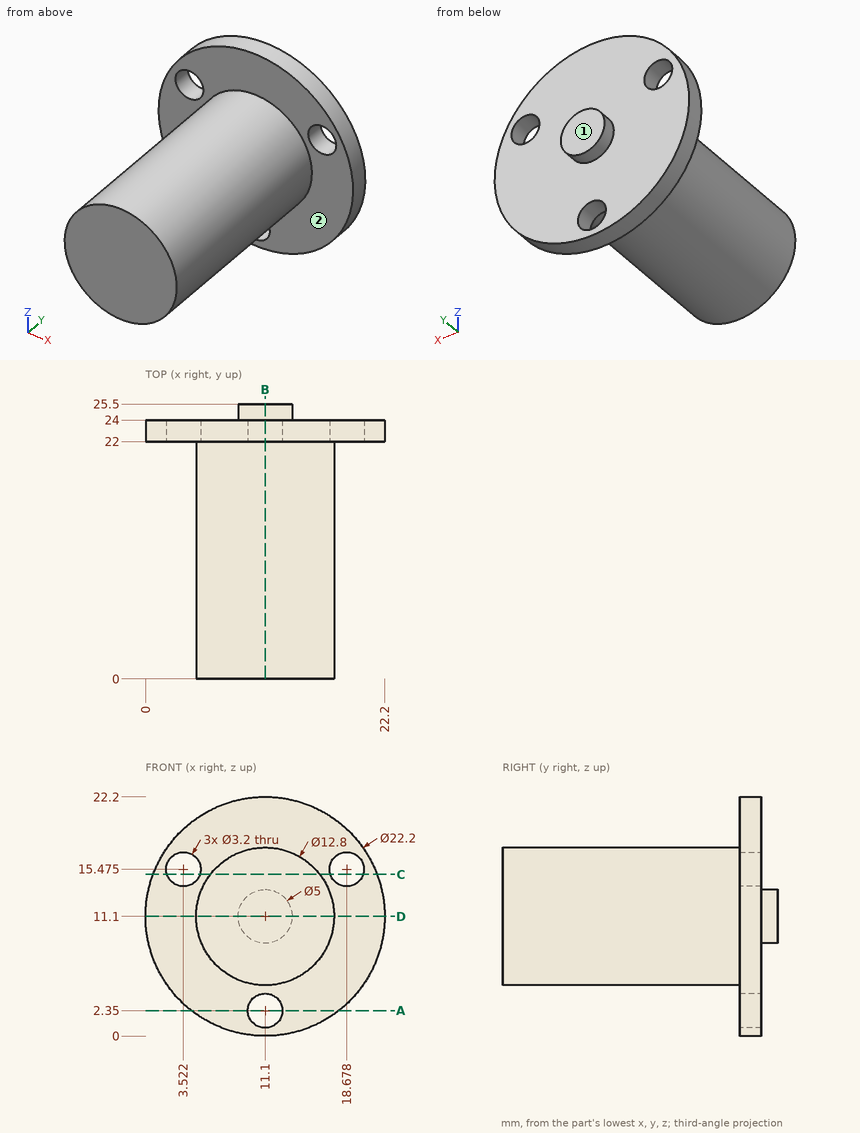
Drawing for the job (mm, zero at the part's lowest x, y, z). A direction names the side the tool comes from. Round coordinates to 2 decimals unless told otherwise and drop trailing zeros. Order: outer loops, then holes, each group sorted by start corner. A loop starts at its lowest first (then second) coordinate and runs counter-clockwise, first axis right, second up. Notation, with made-up numbers: (52, 62) -> (79, 62) arc R22 ccw to (79, 79) -> close; hole circle Ø5 at (85.5, 15.5). An arc over 180 degrees is marked (long way). Write item = value, one per line. Start each with the question number.
(1) Which spindle directions (+Z, -Z, +X, -X, +Y, -Y) get a long thin tool onto all of the face, cutting with end or side? Do the marked faces 1 and 2. Say none if no direction does.
(2) Pin check, flat tips, straight feed: P1, Ø5, axis at y = 23, z = 3.5, coming from the -X side; P2, Ø8, axis at x = 6, z = 16.5, coming from the +Y side; P3, Ø8, axis at y = 12.5, z = 3.5, coming from the +X side. Stop position of each tip, or through.
(3) Probe line 1 (Y direction, x = 8.5, z = 16.5); line 2 (Y direction, x = 16.5, z = 15); line 3 (X direction, y = 19.75, z = 11). List the from-to ranges inside material, lowest first. Write a range as [from, to].
(4) Cut at B-B, the plane x = 11.1. List the corners of the cut face in (y, z).
(5) Cut at D-D, the plane z = 11.1. List the corners of the cut face in (x, y).
(6) Cut at C-C, the plane z = 15. State how many separate pieces and enclosed holes the cut face has, then the cut area to 3 significant figures.
(7) Cut at A-A, the plane z = 2.35. List the corners of the cut face in (x, y), then the cut area to 3 significant figures.
Model answer:
q1.face_1 = +Z, -Z, +X, -X, +Y
q1.face_2 = -Y
q2.P1 = 1.24
q2.P2 = 24
q2.P3 = 16.39
q3.line_1 = [0, 24]
q3.line_2 = [22, 24]
q3.line_3 = [4.7, 17.5]
q4.outline = (0, 4.7) -> (22, 4.7) -> (22, 3.95) -> (24, 3.95) -> (24, 8.6) -> (25.5, 8.6) -> (25.5, 13.6) -> (24, 13.6) -> (24, 22.2) -> (22, 22.2) -> (22, 17.5) -> (0, 17.5) -> close; (22, 0) -> (24, 0) -> (24, 0.75) -> (22, 0.75) -> close
q5.outline = (0, 22) -> (4.7, 22) -> (4.7, 0) -> (17.5, 0) -> (17.5, 22) -> (22.2, 22) -> (22.2, 24) -> (13.6, 24) -> (13.6, 25.5) -> (8.6, 25.5) -> (8.6, 24) -> (0, 24) -> close
q6.separate_pieces = 3
q6.enclosed_holes = 0
q6.area = 253 mm2
q7.outline = (4.27, 22) -> (9.5, 22) -> (9.5, 24) -> (4.27, 24) -> close; (12.7, 22) -> (17.93, 22) -> (17.93, 24) -> (12.7, 24) -> close
q7.area = 20.9 mm2
